Check sheet for the drawn part. Datum: minimum x, y, z corner. Units: mm. A direction names the side the tool comes from. Give positions to 0.01 mm unless a question says otherwise; leave off trailing zeros. Loops run counter-clockwise (first coordinate to the right, second up) from the corner with the lowest first, then second, coordinate; pieces in that order, holes last.
1. Go/stop test with flat-tipped pins: pin 1 Ø8.5 at (x, z) = (33, 58.82) entering from -Y; pin 2 Ø4 at (x, y) = (8, 3.5) entering from -Z; pin 3 Ø3 at (y, z) = (3, 30.5) entering from -X. Record where each tip stops, or that it passes through.
2. Cross-section at C-C, the plane z = 15.5. Record the cut outline in (x, y).
3. Tool access check on the marked faces 1 and 2. Record the directions out of +Z, -Z, +X, -X, +Y, -Y that give a thin tool (end or side, any length) a straight path to the whole face; none if there is none.
4. Cross-section at A-A, the plane z = 33. Record the cut outline in (x, y), plus the area to 3 significant figures.
5. Cross-section at D-D, the plane y = 4.5. Record the cut outline in (x, z), plus the area to 3 significant figures.
6. Material ranges on L1, parallel to Y at x = 25, z = 62; L2, parallel to Z at x = 36, y = 0.5; L3, parallel to Z at x = 39, y = 4, recorded low to high.
7. Cross-section at B-B, the plane x = 40.5. Record the cut outline in (y, z), plus the area to 3 significant figures.
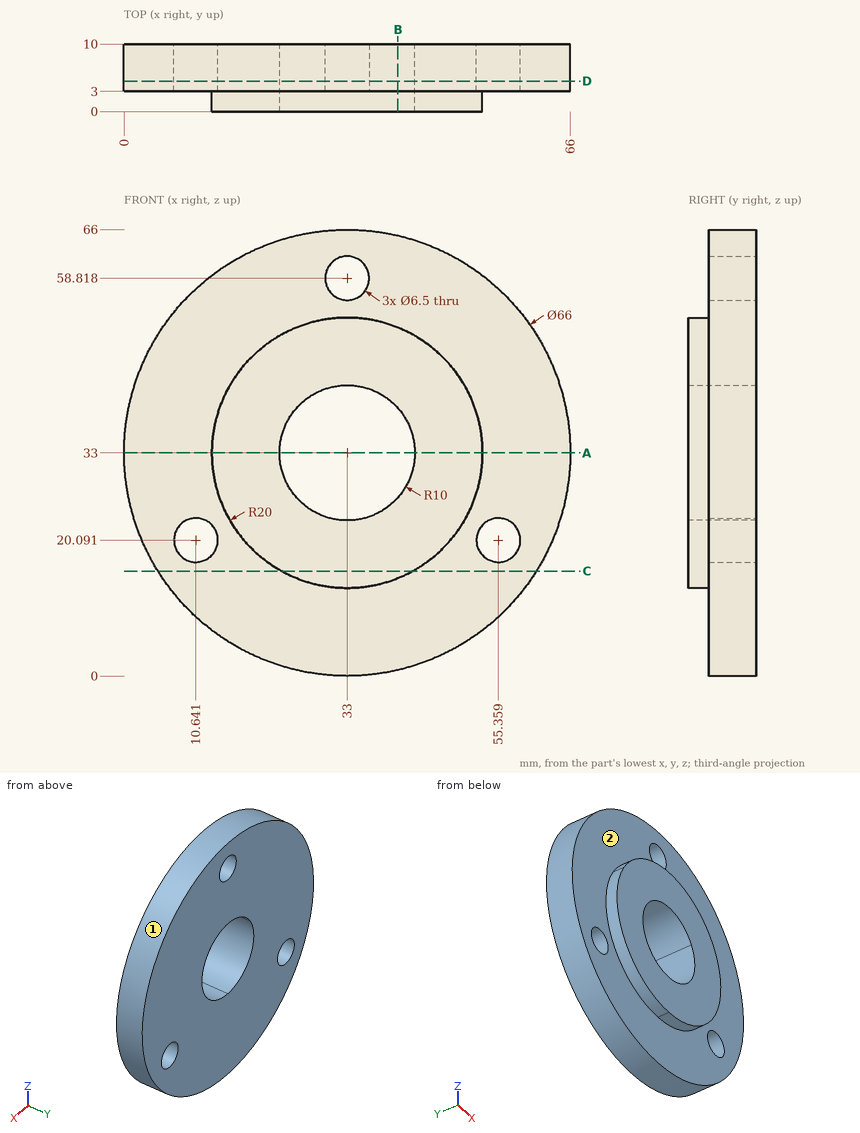
Result:
1. pin 1: stops at y = 3
1. pin 2: stops at z = 9.34
1. pin 3: stops at x = 0.02
2. outline: (5.02, 3) - (23.32, 3) - (23.32, 0) - (42.68, 0) - (42.68, 3) - (60.98, 3) - (60.98, 10) - (5.02, 10) - close
3. face 1: +Y, -Y
3. face 2: -Y
4. outline: (0, 3) - (13, 3) - (13, 0) - (23, 0) - (23, 10) - (0, 10) - close; (43, 0) - (53, 0) - (53, 3) - (66, 3) - (66, 10) - (43, 10) - close
4. area: 382 mm2
5. outline: circle Ø66 at (33, 33); hole circle Ø6.5 at (10.64, 20.09); hole circle Ø20 at (33, 33); hole circle Ø6.5 at (33, 58.82); hole circle Ø6.5 at (55.36, 20.09)
5. area: 3,010 mm2
6. L1: y = 3 to 10
6. L2: z = 13.23 to 23.46, 42.54 to 52.77
6. L3: z = 0.55 to 25, 41 to 65.45
7. outline: (0, 14.46) - (3, 14.46) - (3, 0.86) - (10, 0.86) - (10, 26.39) - (0, 26.39) - close; (0, 39.61) - (10, 39.61) - (10, 65.14) - (3, 65.14) - (3, 51.54) - (0, 51.54) - close
7. area: 429 mm2
